```python
from build123d import *

# Parameters (mm, degrees)
F0_R     = 1.5
F1_DEPTH = 1


with BuildPart() as f1:
    # F0 (on Top) → F1 (new body)
    with BuildSketch(Plane.XY):
        with BuildLine():
            Line((0, -5), (0, 0))
            Line((0, 0), (-6, 0))
            ThreePointArc((-6, 0), (-7.114352, -2.333309), (-9.629555, -2.9332))
            Line((-9.629555, -2.9332), (0, -5))
        make_face()
        with BuildLine():
            Line((-6, 0), (0, 0))
            Line((0, 0), (0, 5))
            Line((0, 5), (-9.629555, 2.9332))
            ThreePointArc((-9.629555, 2.9332), (-7.114352, 2.333309), (-6, 0))
        make_face()
        with BuildLine():
            Line((0, 5), (0, 0))
            Line((0, 0), (6, 0))
            ThreePointArc((6, 0), (7.114352, 2.333309), (9.629555, 2.9332))
            Line((9.629555, 2.9332), (0, 5))
        make_face()
        with BuildLine():
            Line((6, 0), (0, 0))
            Line((0, 0), (0, -5))
            Line((0, -5), (9.629555, -2.9332))
            ThreePointArc((9.629555, -2.9332), (7.114352, -2.333309), (6, 0))
        make_face()
        with BuildLine():
            ThreePointArc((9.629555, 2.9332), (7.114352, 2.333309), (6, 0))
            ThreePointArc((6, 0), (7.114352, -2.333309), (9.629555, -2.9332))
            ThreePointArc((9.629555, -2.9332), (11.333309, -1.885648), (12, 0))
            ThreePointArc((12, 0), (11.333309, 1.885648), (9.629555, 2.9332))
        make_face()
        with BuildLine():
            ThreePointArc((10.5, 0), (9, -1.5), (7.5, 0))
            ThreePointArc((7.5, 0), (9, 1.5), (10.5, 0))
        make_face(mode=Mode.SUBTRACT)
        with BuildLine():
            ThreePointArc((-9.629555, -2.9332), (-7.114352, -2.333309), (-6, 0))
            ThreePointArc((-6, 0), (-7.114352, 2.333309), (-9.629555, 2.9332))
            ThreePointArc((-9.629555, 2.9332), (-12, 0), (-9.629555, -2.9332))
        make_face()
        with Locations((-9, 0)):
            Circle(F0_R, mode=Mode.SUBTRACT)
    extrude(amount=F1_DEPTH)


solid = f1.part
```
Input: part model. Units: mm. Frame: model coordinates. Give positions to 0.01 mm unless a question says otherwise; leave off trailing zeros. Order: outer loops, then holes, each group sorted by start corner. A loop starts at its lowest first (then second) coordinate and runs counter-clockwise, first axis right, second up.
1. Material intervals for L1, parallel to X at y = 0.25, z = 0.45; L2, parallel to Y at x = 8.25, z = 0.2; L3, parallel to X at y = 1, z = 0.2, sorted ascending.
Derived:
L1: x = -11.99 to -10.48, -7.52 to 7.52, 10.48 to 11.99
L2: y = -3.23 to -1.3, 1.3 to 3.23
L3: x = -11.83 to -10.12, -7.88 to 7.88, 10.12 to 11.83
2. Section C-C on x = -9. Return the cut outline in (y, z).
Derived:
outline: (-3.07, 0) - (-1.5, 0) - (-1.5, 1) - (-3.07, 1) - close; (1.5, 0) - (3.07, 0) - (3.07, 1) - (1.5, 1) - close
3. Section B-B on z = 0.8. Return the cut outline in (x, y), and give its area (3 significant figures).
Derived:
outline: (-9.63, -2.93) - (0, -5) - (9.63, -2.93) arc R3 ccw to (12, 0) arc R3 ccw to (9.63, 2.93) - (0, 5) - (-9.63, 2.93) arc R3 ccw to start; hole circle Ø3 at (-9, 0); hole circle Ø3 at (9, 0)
area: 159 mm2
4. Section A-A on y = 1.25. Return the cut outline in (x, z), and give its area (3 significant figures).
Derived:
outline: (-11.73, 0) - (-9.83, 0) - (-9.83, 1) - (-11.73, 1) - close; (-8.17, 0) - (8.17, 0) - (8.17, 1) - (-8.17, 1) - close; (9.83, 0) - (11.73, 0) - (11.73, 1) - (9.83, 1) - close
area: 20.1 mm2
5. Mould query, pull axis Y, two halves, no side actions, for faces 1 (the flat face through (-4.75, 3.98, 0.49)), 2 (the flat face through (0, 0, 0)), 3 (the flat face through (-4.882, -3.952, 0.493)), 4 (the cylindrical face through (-10.5, 0.07, 0.49)). Classes: released by +Y, released by -Y, zero draft, split by the parting line, or undercut.
Derived:
face 1: released by +Y
face 2: zero draft
face 3: released by -Y
face 4: undercut
6. Section D-D on y = -0.25. Return the cut outline in (x, z), and give its area (3 significant figures).
Derived:
outline: (-11.99, 0) - (-10.48, 0) - (-10.48, 1) - (-11.99, 1) - close; (-7.52, 0) - (7.52, 0) - (7.52, 1) - (-7.52, 1) - close; (10.48, 0) - (11.99, 0) - (11.99, 1) - (10.48, 1) - close
area: 18.1 mm2
